from build123d import *

# Parameters (mm, degrees)
SKETCH1_R           = 5
BOSS_EXTRUDE1_DEPTH = 2.5
FILLET1_R           = 0.5
FILLET2_R           = 0.5
SKETCH2_R           = 0.95
BOSS_EXTRUDE2_DEPTH = 2.9
SKETCH3_R           = 5
BOSS_EXTRUDE3_DEPTH = 2.5
FILLET3_R           = 0.5


with BuildPart() as part:
    # Sketch1 → Boss-Extrude1 (new body)
    with BuildSketch(Plane.XY):
        Circle(SKETCH1_R)
    extrude(amount=BOSS_EXTRUDE1_DEPTH)

    # Fillet1
    fillet1_edges = [part.edges().sort_by_distance(p)[0] for p in [
        (-5, 0, 0),
    ]]
    fillet(fillet1_edges, radius=FILLET1_R)

    # Fillet2
    fillet2_edges = [part.edges().sort_by_distance(p)[0] for p in [
        (-5, 0, 2.5),
    ]]
    fillet(fillet2_edges, radius=FILLET2_R)

    # Sketch2 → Boss-Extrude2 (add)
    with BuildSketch(Plane.XY.offset(2.5)):
        Circle(SKETCH2_R)
    extrude(amount=BOSS_EXTRUDE2_DEPTH)

    # Sketch3 → Boss-Extrude3 (add)
    with BuildSketch(Plane.XY.offset(5.4)):
        Circle(SKETCH3_R)
    extrude(amount=BOSS_EXTRUDE3_DEPTH)

    # Fillet3
    fillet3_edges = [part.edges().sort_by_distance(p)[0] for p in [
        (-5, 0, 5.4),
        (-5, 0, 7.9),
    ]]
    fillet(fillet3_edges, radius=FILLET3_R)


solid = part.part
Check sheet for the modelled part. Datum: model origin and axes. Units: mm. A direction names the side the tool comes from. Give positions to 0.01 mm unless a question says otherwise; leave off trailing zeros. Order: outer loops, then holes, each group sorted by start corner. A loop starts at its lowest first (then second) coordinate and runs counter-clockwise, first axis right, second up. Notation, with made-up numbers: M 76.5,62 L 115.5,62 A17 cw 115.5,85 Z; hole C 17.5,10.5 d2. An arc over 180 degrees is marked long. Answer as CSV lines item,"result". Start each with the question number.
Item 1: Mould release check, pull along Z, two halves, no side actions. Record for faces 1 (the face through (0, 0, 7.9)), 2 (the face through (0, 0, 0)), 3 (the face through (-1.1, 0.1, 2.5)): +Z half, -Z half, draft (parallel to the pull), parting line (faces both ways), or undercut.
Item 2: Cross-section at A-A on x = 0. Enter the section's corners in (y, z).
Item 3: Tool access check on faces 4 (the face through (-0.95, 0.04, 3.93)), 5 (the face through (-1.08, -4.88, 6.64)). Record the directions out of +Z, -Z, +X, -X, +Y, -Y that give a thin tool (end or side, any length) a straight path to the whole face; none if there is none.
Item 4: Thickness scan on line 1 (Z direction, x = 2, y = 0); line 2 (Y direction, x = 0, z = 2.75); line 3 (X direction, y = -1.5, z = 2.25). Record the ranges inside material, lowest first. Write a range as [from, to].
Item 5: Cross-section at D-D on z = 1. Enter the section's corners in (x, y).
Item 6: Cross-section at C-C on z = 3. Enter the section's corners in (x, y).
Item 7: Gauge pin test, flat ends, axial feed: P1, Ø6, axis at x = 2, y = -1, coming from the -Z side; P2, Ø1.5, axis at y = 3, z = 3, coming from the -X side; P3, Ø1.5, axis at y = 4, z = 2, coming from the -X side. Record the tip position at first contact, or that the pin passes through.
Established:
1,face 1,"+Z half"
1,face 2,"-Z half"
1,face 3,"undercut"
2,outline,"M -5,0.5 A0.5 ccw -4.5,0 L 4.5,0 A0.5 ccw 5,0.5 L 5,2 A0.5 ccw 4.5,2.5 L 0.95,2.5 L 0.95,5.4 L 4.5,5.4 A0.5 ccw 5,5.9 L 5,7.4 A0.5 ccw 4.5,7.9 L -4.5,7.9 A0.5 ccw -5,7.4 L -5,5.9 A0.5 ccw -4.5,5.4 L -0.95,5.4 L -0.95,2.5 L -4.5,2.5 A0.5 ccw -5,2 Z"
3,face 4,"none"
3,face 5,"+Z, -Z"
4,line 1,"z = [0, 2.5], [5.4, 7.9]"
4,line 2,"y = [-0.95, 0.95]"
4,line 3,"x = [-4.7, 4.7]"
5,outline,"C 0,0 d10"
6,outline,"C 0,0 d1.9"
7,P1,"stops at z = 0"
7,P2,"stops at x = -4.09"
7,P3,"stops at x = -3.8"
